from build123d import *

# Parameters (mm, degrees)
F0_W     = 67
F0_H     = 44
F1_DEPTH = 2
F4_R     = 1.75
F5_DEPTH = 30
F7_DEPTH = 2


with BuildPart() as f1:
    # F0 (on Top) → F1 (new body)
    with BuildSketch(Plane.XY):
        Polygon((-37.5, -21), (-37.5, -26), (-32.5, -26), (-32.5, -25), (-36.5, -25), (-36.5, -21), align=None)
        Polygon((-32.5, -25), (-32.5, -26), (32.5, -26), (32.5, -25), (36.5, -25), (36.5, -21), (37.5, -21), (37.5, 21), (36.5, 21), (36.5, 25), (32.5, 25), (32.5, 26), (-32.5, 26), (-32.5, 25), (-36.5, 25), (-36.5, 21), (-37.5, 21), (-37.5, -21), (-36.5, -21), (-36.5, -25), align=None)
        Rectangle(F0_W, F0_H, mode=Mode.SUBTRACT)
        Polygon((32.5, -25), (32.5, -26), (37.5, -26), (37.5, -21), (36.5, -21), (36.5, -25), align=None)
        Polygon((-37.5, 25), (-37.5, 21), (-36.5, 21), (-36.5, 25), (-32.5, 25), (-32.5, 26), (-36.5, 26), (-37.5, 26), align=None)
        Polygon((36.5, 21), (37.5, 21), (37.5, 25), (37.5, 26), (36.5, 26), (32.5, 26), (32.5, 25), (36.5, 25), align=None)
    extrude(amount=F1_DEPTH)


with BuildPart() as f2_1:
    # F2: copy of F1
    add(f1.part.moved(Location((0, 0, 30))))


with BuildPart() as f3_1:
    # F3: copy of F1
    add(f1.part.moved(Location((0, 0, 15))))


with BuildPart() as f1_1:
    add(f1.part)

    add(f2_1.part)  # F5 merges F2_1

    add(f3_1.part)  # F5 merges F3_1
    # F4 (on Top) → F5 (join)
    with BuildSketch(Plane.XY):
        with Locations((-35.5, 24)):
            Circle(F4_R)
        with Locations((-23.6666666667, 24)):
            Circle(F4_R)
        with Locations((-11.8333333333, 24)):
            Circle(F4_R)
        with Locations((0, 24)):
            Circle(F4_R)
        with Locations((11.8333333333, 24)):
            Circle(F4_R)
        with Locations((23.6666666667, 24)):
            Circle(F4_R)
        with Locations((35.5, 24)):
            Circle(F4_R)
        with Locations((-35.5, 12)):
            Circle(F4_R)
        with Locations((-35.5, 0)):
            Circle(F4_R)
        with Locations((-35.5, -12)):
            Circle(F4_R)
        with Locations((-35.5, -24)):
            Circle(F4_R)
        with Locations((35.5, 12)):
            Circle(F4_R)
        with Locations((35.5, 0)):
            Circle(F4_R)
        with Locations((35.5, -12)):
            Circle(F4_R)
        with Locations((35.5, -24)):
            Circle(F4_R)
        with Locations((-23.6666666667, -24)):
            Circle(F4_R)
        with Locations((-11.8333333333, -24)):
            Circle(F4_R)
        with Locations((0, -24)):
            Circle(F4_R)
        with Locations((11.8333333333, -24)):
            Circle(F4_R)
        with Locations((23.6666666667, -24)):
            Circle(F4_R)
    extrude(amount=F5_DEPTH)

    # F6 (on face) → F7 (join)
    with BuildSketch(Plane(origin=(0, 0, 0), x_dir=(1, 0, 0), z_dir=(0, 0, -1))):
        Polygon((-32.5, 26), (-37.5, 26), (-37.5, 21), (-36.2434542816, 21), (-36.2434542816, 25), (-32.5, 25), align=None)
    extrude(amount=F7_DEPTH)

    # F8: F1 across plane


with BuildPart() as f1_2:
    add(f1_1.part)
    add(f1_1.part.mirror(Plane.YZ))

    # F9: F1 across plane


with BuildPart() as f1_3:
    add(f1_2.part)
    add(f1_2.part.mirror(Plane.XZ))


solid = f1_3.part
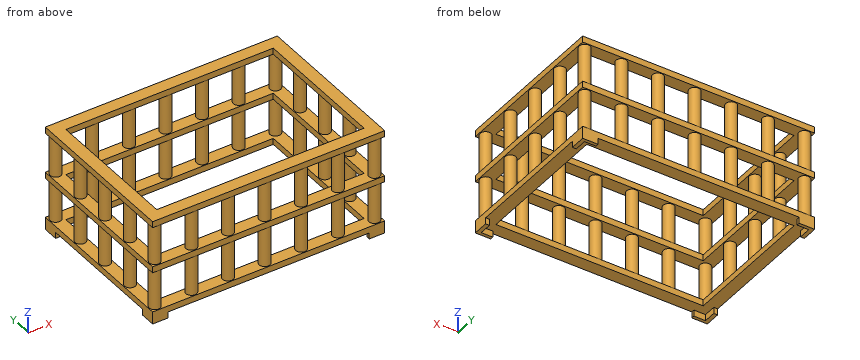
Here's how the part is built. I have some questions about the finished solid (model axes, mm). Coordinates: 2 decimals unless noted, no trailing zeros. Order: outer loops, then holes, each group sorted by start corner. A loop starts at its lowest first (then second) coordinate and runs counter-clockwise, first axis right, second up. Notation, with made-up numbers: (89.5, 35) -> (97.5, 35) arc R24 cw to (97.5, 62) -> close; hole circle Ø6 at (-25, -37.75). An arc over 180 degrees is marked (long way). Answer in a Markdown table with one row per item.
(1) Please list where these lines run through material, in increasing order: probe 1 along Z at (x, y) = (4, 24); probe 2 along Y at (x, z) = (-27, 0.5); probe 3 along X at (y, z) = (-12, 9.5).
Answer key:
| item | result |
|---|---|
| probe 1 | 0 to 2, 15 to 17, 30 to 32 |
| probe 2 | -26 to -22, 22 to 26 |
| probe 3 | -37.25 to -33.75, 33.75 to 37.25 |
(2) Will these pins go through, and if not, where does the flat tip stop? pin 1 Ø5 at (x, z) = (25.5, 23.5) entering from +Y; pin 2 Ø1.5 at (y, z) = (10.5, 20.5) entering from +X; pin 3 Ø10 at (x, y) = (24, -7) entering from -Z.
Answer key:
| item | result |
|---|---|
| pin 1 | y = 25.75 |
| pin 2 | x = 37.08 |
| pin 3 | through |
(3) I want a section at B-B on x = -17. List the corners of the cut face in (y, z) for me.
Answer key:
| item | result |
|---|---|
| outline | (-26, 0) -> (-22, 0) -> (-22, 2) -> (-26, 2) -> close; (-26, 15) -> (-22, 15) -> (-22, 17) -> (-26, 17) -> close; (-26, 30) -> (-22, 30) -> (-22, 32) -> (-26, 32) -> close; (22, 0) -> (26, 0) -> (26, 2) -> (22, 2) -> close; (22, 15) -> (26, 15) -> (26, 17) -> (22, 17) -> close; (22, 30) -> (26, 30) -> (26, 32) -> (22, 32) -> close |
(4) I want a section at A-A on z = 22.5. Count the separate pieces of the cut face and the enclosed holes in it, then the cut area to 3 significant figures.
Answer key:
| item | result |
|---|---|
| separate pieces | 20 |
| enclosed holes | 0 |
| area | 192 mm^2 |
